```python
from build123d import *

# Parameters (mm, degrees)
SKETCH1_W           = 166
SKETCH1_H           = 126
BOSS_EXTRUDE1_DEPTH = 7
BOSS_EXTRUDE2_DEPTH = 15
CUT_EXTRUDE1_REACH  = 107.276
SKETCH4_R           = 1.6
CUT_EXTRUDE2_DEPTH  = 106.275828185
SKETCH5_R           = 4
CUT_EXTRUDE3_DEPTH  = 4
CUT_EXTRUDE4_DEPTH  = 107.498826285
CUT_EXTRUDE5_DEPTH  = 3
CUT_EXTRUDE6_DEPTH  = 2
BOSS_EXTRUDE3_DEPTH = 2


with BuildPart() as part:
    # Sketch1 → Boss-Extrude1 (new body)
    with BuildSketch(Plane(origin=(0, 0, 0), x_dir=(1, 0, 0), z_dir=(0, 1, 0))):
        Rectangle(SKETCH1_W, SKETCH1_H)
    extrude(amount=BOSS_EXTRUDE1_DEPTH)

    # Sketch2 → Boss-Extrude2 (add)
    with BuildSketch(Plane(origin=(0, 7, 0), x_dir=(1, 0, 0), z_dir=(0, 1, 0))):
        Polygon((-83, 63), (-83, 12), (64, 12), (64, -63), (83, -63), (83, 63), align=None)
    extrude(amount=BOSS_EXTRUDE2_DEPTH)

    # Sketch3 → Cut-Extrude1 (cut, up to next)
    with BuildSketch(Plane(origin=(0, 7, 0), x_dir=(1, 0, 0), z_dir=(0, 1, 0)), mode=Mode.PRIVATE) as cut_extrude1_sk1:
        with BuildLine():
            Line((-44.67, -11.18), (-40.47, -11.18))
            ThreePointArc((-40.47, -11.18), (-39.409339828, -11.619339828), (-38.97, -12.68))
            Line((-38.97, -12.68), (-38.97, -46.68))
            ThreePointArc((-38.97, -46.68), (-39.409339828, -47.740660172), (-40.47, -48.18))
            Line((-40.47, -48.18), (-44.67, -48.18))
            ThreePointArc((-44.67, -48.18), (-45.730660172, -47.740660172), (-46.17, -46.68))
            Line((-46.17, -46.68), (-46.17, -12.68))
            ThreePointArc((-46.17, -12.68), (-45.730660172, -11.619339828), (-44.67, -11.18))
        make_face()
    cut_extrude1_tool1 = extrude(cut_extrude1_sk1.sketch, amount=-CUT_EXTRUDE1_REACH, mode=Mode.PRIVATE) & part.part
    # Sketch3 → Cut-Extrude1 (cut, up to next)
    with BuildSketch(Plane(origin=(0, 7, 0), x_dir=(1, 0, 0), z_dir=(0, 1, 0)), mode=Mode.PRIVATE) as cut_extrude1_sk2:
        with BuildLine():
            Line((22.89, -11.19), (27.09, -11.19))
            ThreePointArc((27.09, -11.19), (28.150660172, -11.629339828), (28.59, -12.69))
            Line((28.59, -12.69), (28.59, -46.69))
            ThreePointArc((28.59, -46.69), (28.150660172, -47.750660172), (27.09, -48.19))
            Line((27.09, -48.19), (22.89, -48.19))
            ThreePointArc((22.89, -48.19), (21.829339828, -47.750660172), (21.39, -46.69))
            Line((21.39, -46.69), (21.39, -12.69))
            ThreePointArc((21.39, -12.69), (21.829339828, -11.629339828), (22.89, -11.19))
        make_face()
    cut_extrude1_tool2 = extrude(cut_extrude1_sk2.sketch, amount=-CUT_EXTRUDE1_REACH, mode=Mode.PRIVATE) & part.part
    add(cut_extrude1_tool1.solids().sort_by_distance((-42.57, 7, 29.68))[0], mode=Mode.SUBTRACT)
    add(cut_extrude1_tool2.solids().sort_by_distance((24.99, 7, 29.69))[0], mode=Mode.SUBTRACT)

    # Sketch4 → Cut-Extrude2 (cut, through all)
    with BuildSketch(Plane(origin=(0, 7, 0), x_dir=(1, 0, 0), z_dir=(0, 1, 0))):
        with Locations(Location((-76.1, -56.1, 0), (0, 0, 270))):
            Circle(SKETCH4_R)
        with Locations(Location((-20.22, -56.1, 0), (0, 0, 270))):
            Circle(SKETCH4_R)
        with Locations(Location((2.64, -56.1, 0), (0, 0, 270))):
            Circle(SKETCH4_R)
        with Locations(Location((58.49, -56.1, 0), (0, 0, 270))):
            Circle(SKETCH4_R)
        with Locations(Location((-76.1, 6.13, 0), (0, 0, 270))):
            Circle(SKETCH4_R)
        with Locations(Location((-30.38, -4.03, 0), (0, 0, 270))):
            Circle(SKETCH4_R)
        with Locations(Location((58.52, 6.16, 0), (0, 0, 270))):
            Circle(SKETCH4_R)
        with Locations(Location((12.8, -4, 0), (0, 0, 270))):
            Circle(SKETCH4_R)
    extrude(amount=-CUT_EXTRUDE2_DEPTH, mode=Mode.SUBTRACT)

    # Sketch5 → Cut-Extrude3 (cut)
    with BuildSketch(Plane(origin=(0, 0, 0), x_dir=(-1, 0, 0), z_dir=(0, -1, 0))):
        with BuildLine():
            Line((70.6, -58), (25.705435261, -58))
            ThreePointArc((25.705435261, -58), (24.606882494, -57.521362726), (24.209407462, -56.390909091))
            ThreePointArc((24.209407462, -56.390909091), (20.22, -52.1), (16.230592538, -56.390909091))
            ThreePointArc((16.230592538, -56.390909091), (15.833117506, -57.521362726), (14.734564739, -58))
            Line((14.734564739, -58), (2.845435261, -58))
            ThreePointArc((2.845435261, -58), (1.746882494, -57.521362726), (1.349407462, -56.390909091))
            ThreePointArc((1.349407462, -56.390909091), (-2.64, -52.1), (-6.629407462, -56.390909091))
            ThreePointArc((-6.629407462, -56.390909091), (-7.026882494, -57.521362726), (-8.125435261, -58))
            Line((-8.125435261, -58), (-53.004564739, -58))
            ThreePointArc((-53.004564739, -58), (-54.103117506, -57.521362726), (-54.500592538, -56.390909091))
            ThreePointArc((-54.500592538, -56.390909091), (-58.49, -52.1), (-62.479407462, -56.390909091))
            ThreePointArc((-62.479407462, -56.390909091), (-62.876882494, -57.521362726), (-63.975435261, -58))
            Line((-63.975435261, -58), (-76.5, -58))
            ThreePointArc((-76.5, -58), (-77.560660172, -57.560660172), (-78, -56.5))
            Line((-78, -56.5), (-78, 56.5))
            ThreePointArc((-78, 56.5), (-77.560660172, 57.560660172), (-76.5, 58))
            Line((-76.5, 58), (76.5, 58))
            ThreePointArc((76.5, 58), (77.560660172, 57.560660172), (78, 56.5))
            Line((78, 56.5), (78, 11.615435261))
            ThreePointArc((78, 11.615435261), (77.521362726, 10.516882494), (76.390909091, 10.119407462))
            ThreePointArc((76.390909091, 10.119407462), (72.1, 6.13), (76.390909091, 2.140592538))
            ThreePointArc((76.390909091, 2.140592538), (77.521362726, 1.743117506), (78, 0.644564739))
            Line((78, 0.644564739), (78, -50.6))
            ThreePointArc((78, -50.6), (77.560660172, -51.660660172), (76.5, -52.1))
            Line((76.5, -52.1), (76.1, -52.1))
            ThreePointArc((76.1, -52.1), (73.271572875, -53.271572875), (72.1, -56.1))
            Line((72.1, -56.1), (72.1, -56.5))
            ThreePointArc((72.1, -56.5), (71.660660172, -57.560660172), (70.6, -58))
        make_face()
        with Locations(Location((30.38, -4.03, 0), (0, 0, 90))):
            Circle(SKETCH5_R, mode=Mode.SUBTRACT)
        with Locations(Location((-12.8, -4, 0), (0, 0, 90))):
            Circle(SKETCH5_R, mode=Mode.SUBTRACT)
        with Locations(Location((-58.52, 6.16, 0), (0, 0, 90))):
            Circle(SKETCH5_R, mode=Mode.SUBTRACT)
    extrude(amount=-CUT_EXTRUDE3_DEPTH, mode=Mode.SUBTRACT)

    # Sketch6 → Cut-Extrude4 (cut, through all)
    with BuildSketch(Plane(origin=(0, 22, 0), x_dir=(1, 0, 0), z_dir=(0, 1, 0))):
        with BuildLine():
            Line((25.2, 56.05), (49.2, 56.05))
            ThreePointArc((49.2, 56.05), (50.260660172, 55.610660172), (50.7, 54.55))
            Line((50.7, 54.55), (50.7, 47.55))
            ThreePointArc((50.7, 47.55), (50.260660172, 46.489339828), (49.2, 46.05))
            Line((49.2, 46.05), (25.2, 46.05))
            ThreePointArc((25.2, 46.05), (24.139339828, 46.489339828), (23.7, 47.55))
            Line((23.7, 47.55), (23.7, 54.55))
            ThreePointArc((23.7, 54.55), (24.139339828, 55.610660172), (25.2, 56.05))
        make_face()
    extrude(amount=-CUT_EXTRUDE4_DEPTH, mode=Mode.SUBTRACT)

    # Sketch7 → Cut-Extrude5 (cut)
    with BuildSketch(Plane.XZ.offset(-4)):
        with BuildLine():
            Line((-27.5, -56), (-59.5, -56))
            ThreePointArc((-59.5, -56), (-60.560660172, -55.560660172), (-61, -54.5))
            Line((-61, -54.5), (-61, -27.5))
            ThreePointArc((-61, -27.5), (-60.560660172, -26.439339828), (-59.5, -26))
            Line((-59.5, -26), (-27.5, -26))
            ThreePointArc((-27.5, -26), (-26.439339828, -26.439339828), (-26, -27.5))
            Line((-26, -27.5), (-26, -54.5))
            ThreePointArc((-26, -54.5), (-26.439339828, -55.560660172), (-27.5, -56))
        make_face()
    extrude(amount=-CUT_EXTRUDE5_DEPTH, mode=Mode.SUBTRACT)

    # Sketch8 → Cut-Extrude6 (cut)
    with BuildSketch(Plane.XZ.offset(-4)):
        with BuildLine():
            Line((55.3, 45.9), (64.3, 45.9))
            ThreePointArc((64.3, 45.9), (65.360660172, 45.460660172), (65.8, 44.4))
            Line((65.8, 44.4), (65.8, 29.4))
            ThreePointArc((65.8, 29.4), (65.360660172, 28.339339828), (64.3, 27.9))
            Line((64.3, 27.9), (55.3, 27.9))
            ThreePointArc((55.3, 27.9), (54.239339828, 28.339339828), (53.8, 29.4))
            Line((53.8, 29.4), (53.8, 44.4))
            ThreePointArc((53.8, 44.4), (54.239339828, 45.460660172), (55.3, 45.9))
        make_face()
    extrude(amount=-CUT_EXTRUDE6_DEPTH, mode=Mode.SUBTRACT)

    # Sketch9 → Boss-Extrude3 (add)
    with BuildSketch(Plane(origin=(0, 4, 0), x_dir=(-1, 0, 0), z_dir=(0, -1, 0))):
        with BuildLine():
            Line((-8.082795796, -11.112795796), (6.059339828, 3.029339828))
            ThreePointArc((6.059339828, 3.029339828), (7.12, 3.468679656), (8.180660172, 3.029339828))
            Line((8.180660172, 3.029339828), (22.322795796, -11.112795796))
            ThreePointArc((22.322795796, -11.112795796), (22.762135624, -12.173455967), (22.322795796, -13.234116139))
            Line((22.322795796, -13.234116139), (8.180660172, -27.376251763))
            ThreePointArc((8.180660172, -27.376251763), (7.12, -27.815591591), (6.059339828, -27.376251763))
            Line((6.059339828, -27.376251763), (-8.082795796, -13.234116139))
            ThreePointArc((-8.082795796, -13.234116139), (-8.522135624, -12.173455967), (-8.082795796, -11.112795796))
        make_face()
    extrude(amount=BOSS_EXTRUDE3_DEPTH)


solid = part.part
```
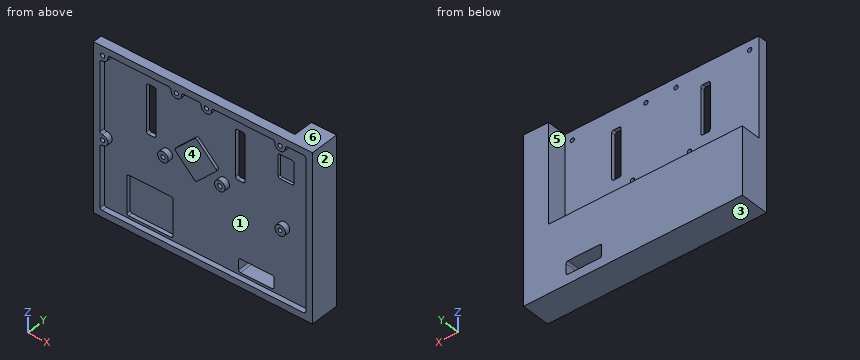
Check sheet for the modelled part. Datum: model origin and axes. Units: mm. Face numbers are marked on the shaded views. A direction names the side the tool comes from. Round coordinates to 2 decimals unless told otherwise and drop trailing zeros. Order: outer loops, then holes, each group sorted by start corner. A loop starts at its lowest first (then second) coordinate and runs counter-clockwise, first axis right, second up. Notation, with made-up numbers: (81, 36.5) - (137, 36.5) arc R14 ccw to (137, 40.5) - close; hole circle Ø5 at (48.25, 21). An arc over 180 degrees is marked (long way). Answer as CSV lines item,"result". Start each with the question number.
1) Section check B-B (y = 9.25). Record the cut outline in (x, z), then the cut area to 3 significant figures.
2) Section check C-C (z = -34). Record the cut outline in (x, y).
3) Scan lines: probe 1 along X at (y, z) = (4.25, 56.1); probe 2 along X at (y, z) = (4.5, -6.13); probe 3 along Z at (x, y) = (23, 5.25). Record each from-to range of solid material in increasing order.
4) Section check D-D (z = 23). Record the cut outline in (x, y).
5) Tool access check on the marked faces 4, 5 and 6. Record the directions out of +Z, -Z, +X, -X, +Y, -Y that give a thin tool (end or side, any length) a straight path to the whole face; none if there is none.
6) Draft check along X on the marked faces 1, 2 and 3. Enter one of: +X half, -X half, draft (parallel to the pull), parting line (faces both ways), or undercut.
7) Depth check by flat-ended pin: pin 1 (4 mm diameter, centred on x = 60, z = 4, fed in from +Y); pin 2 (1.5 mm diameter, centred on x = -31.5, y = 9.5, fed in from +Z). Enter the tip coordinate at first touch or a pass-through.
8) Section check A-A (z = -51). Record the cut outline in (x, y).
Determined:
1,outline,"(-83, -63) - (83, -63) - (83, 63) - (64, 63) - (64, -12) - (-83, -12) - close; hole (23.7, -54.55) arc R1.5 ccw to (25.2, -56.05) - (49.2, -56.05) arc R1.5 ccw to (50.7, -54.55) - (50.7, -47.55) arc R1.5 ccw to (49.2, -46.05) - (25.2, -46.05) arc R1.5 ccw to (23.7, -47.55) - close"
1,area,"9,620 mm^2"
2,outline,"(-83, 0) - (-78, 0) - (-78, 4) - (-61, 4) - (-61, 7) - (-26, 7) - (-26, 4) - (78, 4) - (78, 0) - (83, 0) - (83, 22) - (-83, 22) - close"
3,probe 1,"-83 to -77.7, -74.5 to -21.82, -18.62 to 1.04, 4.24 to 56.89, 60.09 to 83"
3,probe 2,"-83 to -77.7, -74.5 to 56.92, 60.12 to 83"
3,probe 3,"-63 to 11.19, 48.19 to 63"
4,outline,"(-83, 0) - (-78, 0) - (-78, 4) - (-46.17, 4) - (-46.17, 7) - (-83, 7) - close; (-38.97, 4) - (-12.56, 4) - (-12.56, 2) - (-1.68, 2) - (-1.68, 4) - (21.39, 4) - (21.39, 7) - (-38.97, 7) - close; (28.59, 4) - (78, 4) - (78, 0) - (83, 0) - (83, 22) - (64, 22) - (64, 7) - (28.59, 7) - close"
5,face 4,"-Y"
5,face 5,"+Z, -X, +Y"
5,face 6,"+Z, +X, -X, +Y, -Y"
6,face 1,"undercut"
6,face 2,"+X half"
6,face 3,"draft"
7,pin 1,"y = 7"
7,pin 2,"z = -12"
8,outline,"(-83, 0) - (-78, 0) - (-78, 4) - (-61, 4) - (-61, 7) - (-26, 7) - (-26, 4) - (23.7, 4) - (23.7, 22) - (-83, 22) - close; (50.7, 4) - (78, 4) - (78, 0) - (83, 0) - (83, 22) - (50.7, 22) - close"
